Input: part model. Units: mm. Frame: model coordinates. Give positions to 0.01 mm unless a question says otherwise; leave off trailing zeros. Loops run counter-clockwise (first coordinate to the right, second up) from the corner with the lowest first, then second, coordinate; pieces in that order, holes last. Notation, with made-up numbers: (7.25, 39) - (64.25, 39) arc R23 ccw to (64.25, 70) - close; hole circle Ø2 at (-35.5, -3). An arc over 180 degrees is marked (long way). Answer as a JSON object with one key per item and string values. Group by question number.
(1) Material intervals for L1, parallel to X at y = 171.5, z = 25.5; L2, parallel to Y at x = 82, z = -32.5; L3, parallel to Y at x = 37.5, z = -24 (3 decimals), sorted ascending.
(2) Section query B-B (x = 30). Count the separate pieces of the cut face and the enclosed holes in it, plus the area to 3 significant figures.
(3) Section query C-C (z = 24.5). Return loops of the section in (x, y), plus the area to 3 significant figures.
(4) Pin query (flat end, axial travel): P1, Ø3, axis at x = 77.5, z = 46.5, coming from the -Y side; P2, Ø2, axis at x = 74.5, z = -13.5, coming from the -Y side; P3, Ø4, axis at y = 167, z = 25.5, coming from the -X side; P4, Ø3, axis at x = 54, z = 9, coming from the +Y side. Return the tip coordinate at first contact, or that it passes through.
(5) Section query A-A (z = -11.5). Return loops of the section in (x, y).
```python
from build123d import *

# Parameters (mm, degrees)
SKETCH2_R                 = 180
SKETCH2_R_2               = 178
EXTRUDE_THIN1_DEPTH       = 90
WRAP1_SECTION_W           = 3
WRAP1_SECTION_H           = 2.3866999
WRAP1_ANGLE               = 41.69859509
WRAP1_SECTOR_2_SECTION_W  = 3
WRAP1_SECTOR_2_SECTION_H  = 85
WRAP1_SECTOR_2_ANGLE      = 2.067873213
WRAP1_SECTOR_3_SECTION_W  = 3
WRAP1_SECTOR_3_SECTION_H  = 85
WRAP1_SECTOR_3_ANGLE      = 1.591549431
WRAP1_SECTOR_4_SECTION_W  = 3
WRAP1_SECTOR_4_SECTION_H  = 85
WRAP1_SECTOR_4_ANGLE      = 1.591549431
WRAP1_SECTOR_5_SECTION_W  = 3
WRAP1_SECTOR_5_SECTION_H  = 85
WRAP1_SECTOR_5_ANGLE      = 1.591549431
WRAP1_SECTOR_6_SECTION_W  = 3
WRAP1_SECTOR_6_SECTION_H  = 85
WRAP1_SECTOR_6_ANGLE      = 1.591549431
WRAP1_SECTOR_7_SECTION_W  = 3
WRAP1_SECTOR_7_SECTION_H  = 85
WRAP1_SECTOR_7_ANGLE      = 1.591549431
WRAP1_SECTOR_8_SECTION_W  = 3
WRAP1_SECTOR_8_SECTION_H  = 85
WRAP1_SECTOR_8_ANGLE      = 1.591549431
WRAP1_SECTOR_9_SECTION_W  = 3
WRAP1_SECTOR_9_SECTION_H  = 85
WRAP1_SECTOR_9_ANGLE      = 1.591549431
WRAP1_SECTOR_10_SECTION_W = 3
WRAP1_SECTOR_10_SECTION_H = 85
WRAP1_SECTOR_10_ANGLE     = 1.591549431
WRAP1_SECTOR_11_SECTION_W = 3
WRAP1_SECTOR_11_SECTION_H = 85
WRAP1_SECTOR_11_ANGLE     = 1.591549431
WRAP1_SECTOR_12_SECTION_W = 3
WRAP1_SECTOR_12_SECTION_H = 85
WRAP1_SECTOR_12_ANGLE     = 1.591549431
WRAP1_SECTOR_13_SECTION_W = 3
WRAP1_SECTOR_13_SECTION_H = 85
WRAP1_SECTOR_13_ANGLE     = 1.591549431
WRAP1_SECTOR_14_SECTION_W = 3
WRAP1_SECTOR_14_SECTION_H = 85
WRAP1_SECTOR_14_ANGLE     = 1.591549431
WRAP1_SECTOR_15_SECTION_W = 3
WRAP1_SECTOR_15_SECTION_H = 85
WRAP1_SECTOR_15_ANGLE     = 1.591549431
WRAP1_SECTOR_16_SECTION_W = 3
WRAP1_SECTOR_16_SECTION_H = 85
WRAP1_SECTOR_16_ANGLE     = 1.115225649
WRAP1_SECTOR_17_SECTION_W = 3
WRAP1_SECTOR_17_SECTION_H = 2.4233001
WRAP1_SECTOR_17_ANGLE     = 41.69859509
SKETCH5_R                 = 180
CUT_EXTRUDE1_DEPTH        = 119


with BuildPart() as part:
    # Sketch2 → Extrude-Thin1 (new body)
    with BuildSketch(Plane(origin=(0, 0, 0), x_dir=(0, 0, -1), z_dir=(1, 0, 0))):
        with Locations((0, -8.237834894)):
            Circle(SKETCH2_R)
        with Locations((0, -8.237834894)):
            Circle(SKETCH2_R_2, mode=Mode.SUBTRACT)
    extrude(amount=EXTRUDE_THIN1_DEPTH)

    # Wrap1 section (on wrap section) → Wrap1 (revolve)
    with BuildSketch(Plane(origin=(0, -8.237834894, 0), x_dir=(0, 0.9080540786996547, 0.41885294574220344), z_dir=(0, -0.41885294574220344, 0.9080540786996547))):
        with Locations((181.5, -88.70726195)):
            Rectangle(WRAP1_SECTION_W, WRAP1_SECTION_H)
    revolve(axis=Axis((0, -8.237834894, 0), (-1, 0, 0)), revolution_arc=WRAP1_ANGLE)

    # Wrap1 sector 2 section (on wrap section) → Wrap1 sector 2 (revolve)
    with BuildSketch(Plane(origin=(0, -8.237834894, 0), x_dir=(0, 0.9080540786996547, 0.41885294574220344), z_dir=(0, -0.41885294574220344, 0.9080540786996547))):
        with Locations((181.5, -45.013912)):
            Rectangle(WRAP1_SECTOR_2_SECTION_W, WRAP1_SECTOR_2_SECTION_H)
    revolve(axis=Axis((0, -8.237834894, 0), (-1, 0, 0)), revolution_arc=WRAP1_SECTOR_2_ANGLE)

    # Wrap1 sector 3 section (on wrap section) → Wrap1 sector 3 (revolve)
    with BuildSketch(Plane(origin=(0, -8.237834894, 0), x_dir=(0, 0.9309215245835882, 0.3652192698461676), z_dir=(0, -0.3652192698461676, 0.9309215245835882))):
        with Locations((181.5, -45.013912)):
            Rectangle(WRAP1_SECTOR_3_SECTION_W, WRAP1_SECTOR_3_SECTION_H)
    revolve(axis=Axis((0, -8.237834894, 0), (-1, 0, 0)), revolution_arc=WRAP1_SECTOR_3_ANGLE)

    # Wrap1 sector 4 section (on wrap section) → Wrap1 sector 4 (revolve)
    with BuildSketch(Plane(origin=(0, -8.237834894, 0), x_dir=(0, 0.9480114707936929, 0.3182361564052382), z_dir=(0, -0.3182361564052382, 0.9480114707936929))):
        with Locations((181.5, -45.013912)):
            Rectangle(WRAP1_SECTOR_4_SECTION_W, WRAP1_SECTOR_4_SECTION_H)
    revolve(axis=Axis((0, -8.237834894, 0), (-1, 0, 0)), revolution_arc=WRAP1_SECTOR_4_ANGLE)

    # Wrap1 sector 5 section (on wrap section) → Wrap1 sector 5 (revolve)
    with BuildSketch(Plane(origin=(0, -8.237834894, 0), x_dir=(0, 0.9627318820416432, 0.2704576183074822), z_dir=(0, -0.2704576183074822, 0.9627318820416432))):
        with Locations((181.5, -45.013912)):
            Rectangle(WRAP1_SECTOR_5_SECTION_W, WRAP1_SECTOR_5_SECTION_H)
    revolve(axis=Axis((0, -8.237834894, 0), (-1, 0, 0)), revolution_arc=WRAP1_SECTOR_5_ANGLE)

    # Wrap1 sector 6 section (on wrap section) → Wrap1 sector 6 (revolve)
    with BuildSketch(Plane(origin=(0, -8.237834894, 0), x_dir=(0, 0.9750459649655612, 0.22200307701556227), z_dir=(0, -0.22200307701556227, 0.9750459649655612))):
        with Locations((181.5, -45.013912)):
            Rectangle(WRAP1_SECTOR_6_SECTION_W, WRAP1_SECTOR_6_SECTION_H)
    revolve(axis=Axis((0, -8.237834894, 0), (-1, 0, 0)), revolution_arc=WRAP1_SECTOR_6_ANGLE)

    # Wrap1 sector 7 section (on wrap section) → Wrap1 sector 7 (revolve)
    with BuildSketch(Plane(origin=(0, -8.237834894, 0), x_dir=(0, 0.9849229407711876, 0.17299364364807088), z_dir=(0, -0.17299364364807088, 0.9849229407711876))):
        with Locations((181.5, -45.013912)):
            Rectangle(WRAP1_SECTOR_7_SECTION_W, WRAP1_SECTOR_7_SECTION_H)
    revolve(axis=Axis((0, -8.237834894, 0), (-1, 0, 0)), revolution_arc=WRAP1_SECTOR_7_ANGLE)

    # Wrap1 sector 8 section (on wrap section) → Wrap1 sector 8 (revolve)
    with BuildSketch(Plane(origin=(0, -8.237834894, 0), x_dir=(0, 0.9923381221628379, 0.1235518162648073), z_dir=(0, -0.1235518162648073, 0.9923381221628379))):
        with Locations((181.5, -45.013912)):
            Rectangle(WRAP1_SECTOR_8_SECTION_W, WRAP1_SECTOR_8_SECTION_H)
    revolve(axis=Axis((0, -8.237834894, 0), (-1, 0, 0)), revolution_arc=WRAP1_SECTOR_8_ANGLE)

    # Wrap1 sector 9 section (on wrap section) → Wrap1 sector 9 (revolve)
    with BuildSketch(Plane(origin=(0, -8.237834894, 0), x_dir=(0, 0.9972729750487846, 0.07380117368542383), z_dir=(0, -0.07380117368542383, 0.9972729750487846))):
        with Locations((181.5, -45.013912)):
            Rectangle(WRAP1_SECTOR_9_SECTION_W, WRAP1_SECTOR_9_SECTION_H)
    revolve(axis=Axis((0, -8.237834894, 0), (-1, 0, 0)), revolution_arc=WRAP1_SECTOR_9_ANGLE)

    # Wrap1 sector 10 section (on wrap section) → Wrap1 sector 10 (revolve)
    with BuildSketch(Plane(origin=(0, -8.237834894, 0), x_dir=(0, 0.9997151648668349, 0.02386606660673497), z_dir=(0, -0.02386606660673497, 0.9997151648668349))):
        with Locations((181.5, -45.013912)):
            Rectangle(WRAP1_SECTOR_10_SECTION_W, WRAP1_SECTOR_10_SECTION_H)
    revolve(axis=Axis((0, -8.237834894, 0), (-1, 0, 0)), revolution_arc=WRAP1_SECTOR_10_ANGLE)

    # Wrap1 sector 11 section (on wrap section) → Wrap1 sector 11 (revolve)
    with BuildSketch(Plane(origin=(0, -8.237834894, 0), x_dir=(0, 0.9996585874143112, -0.02612869320926344), z_dir=(0, 0.02612869320926344, 0.9996585874143112))):
        with Locations((181.5, -45.013912)):
            Rectangle(WRAP1_SECTOR_11_SECTION_W, WRAP1_SECTOR_11_SECTION_H)
    revolve(axis=Axis((0, -8.237834894, 0), (-1, 0, 0)), revolution_arc=WRAP1_SECTOR_11_ANGLE)

    # Wrap1 sector 12 section (on wrap section) → Wrap1 sector 12 (revolve)
    with BuildSketch(Plane(origin=(0, -8.237834894, 0), x_dir=(0, 0.9971033841053801, -0.07605814489979906), z_dir=(0, 0.07605814489979906, 0.9971033841053801))):
        with Locations((181.5, -45.013912)):
            Rectangle(WRAP1_SECTOR_12_SECTION_W, WRAP1_SECTOR_12_SECTION_H)
    revolve(axis=Axis((0, -8.237834894, 0), (-1, 0, 0)), revolution_arc=WRAP1_SECTOR_12_ANGLE)

    # Wrap1 sector 13 section (on wrap section) → Wrap1 sector 13 (revolve)
    with BuildSketch(Plane(origin=(0, -8.237834894, 0), x_dir=(0, 0.9920559416175896, -0.12579749083840142), z_dir=(0, 0.12579749083840142, 0.9920559416175896))):
        with Locations((181.5, -45.013912)):
            Rectangle(WRAP1_SECTOR_13_SECTION_W, WRAP1_SECTOR_13_SECTION_H)
    revolve(axis=Axis((0, -8.237834894, 0), (-1, 0, 0)), revolution_arc=WRAP1_SECTOR_13_ANGLE)

    # Wrap1 sector 14 section (on wrap section) → Wrap1 sector 14 (revolve)
    with BuildSketch(Plane(origin=(0, -8.237834894, 0), x_dir=(0, 0.984528875928502, -0.17522240856397442), z_dir=(0, 0.17522240856397442, 0.984528875928502))):
        with Locations((181.5, -45.013912)):
            Rectangle(WRAP1_SECTOR_14_SECTION_W, WRAP1_SECTOR_14_SECTION_H)
    revolve(axis=Axis((0, -8.237834894, 0), (-1, 0, 0)), revolution_arc=WRAP1_SECTOR_14_ANGLE)

    # Wrap1 sector 15 section (on wrap section) → Wrap1 sector 15 (revolve)
    with BuildSketch(Plane(origin=(0, -8.237834894, 0), x_dir=(0, 0.97454100078232, -0.22420936152220386), z_dir=(0, 0.22420936152220386, 0.97454100078232))):
        with Locations((181.5, -45.013912)):
            Rectangle(WRAP1_SECTOR_15_SECTION_W, WRAP1_SECTOR_15_SECTION_H)
    revolve(axis=Axis((0, -8.237834894, 0), (-1, 0, 0)), revolution_arc=WRAP1_SECTOR_15_ANGLE)

    # Wrap1 sector 16 section (on wrap section) → Wrap1 sector 16 (revolve)
    with BuildSketch(Plane(origin=(0, -8.237834894, 0), x_dir=(0, 0.9621172806653241, -0.27263590784260605), z_dir=(0, 0.27263590784260605, 0.9621172806653241))):
        with Locations((181.5, -45.013912)):
            Rectangle(WRAP1_SECTOR_16_SECTION_W, WRAP1_SECTOR_16_SECTION_H)
    revolve(axis=Axis((0, -8.237834894, 0), (-1, 0, 0)), revolution_arc=WRAP1_SECTOR_16_ANGLE)

    # Wrap1 sector 17 section (on wrap section) → Wrap1 sector 17 (revolve)
    with BuildSketch(Plane(origin=(0, -8.237834894, 0), x_dir=(0, 0.9080540786996547, 0.41885294574220344), z_dir=(0, -0.41885294574220344, 0.9080540786996547))):
        with Locations((181.5, -1.30226195)):
            Rectangle(WRAP1_SECTOR_17_SECTION_W, WRAP1_SECTOR_17_SECTION_H)
    revolve(axis=Axis((0, -8.237834894, 0), (-1, 0, 0)), revolution_arc=WRAP1_SECTOR_17_ANGLE)

    # Sketch5 → Cut-Extrude1 (cut)
    with BuildSketch(Plane(origin=(0, 0, 0), x_dir=(0, 0, -1), z_dir=(1, 0, 0))):
        with Locations((0, -8.237834894)):
            Circle(SKETCH5_R)
    extrude(amount=CUT_EXTRUDE1_DEPTH, mode=Mode.SUBTRACT)


solid = part.part
```
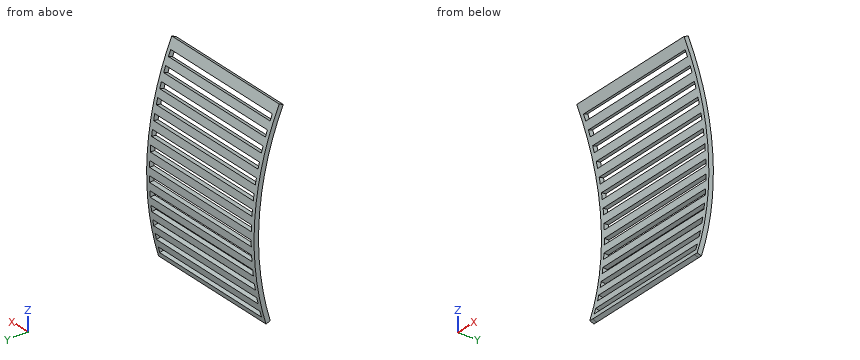
Recorded:
{
 "1": {"L1": "x = 0.09 to 2.51, 87.51 to 89.9", "L2": "y = 168.8 to 171.85", "L3": "y = 170.155 to 173.182"},
 "2": {"separate pieces": "15", "enclosed holes": "0", "area": "227 mm^2"},
 "3": {"outline": "(0.09, 170.09) - (2.51, 170.09) - (2.51, 173.11) - (0.09, 173.11) - close; (87.51, 170.09) - (89.9, 170.09) - (89.9, 173.11) - (87.51, 173.11) - close", "area": "14.6 mm^2"},
 "4": {"P1": "stops at y = 165.24", "P2": "stops at y = 171.18", "P3": "passes through", "P4": "stops at y = 174.57"},
 "5": {"outline": "(0.09, 171.39) - (2.51, 171.39) - (2.51, 174.4) - (0.09, 174.4) - close; (87.51, 171.39) - (89.9, 171.39) - (89.9, 174.4) - (87.51, 174.4) - close"}
}
